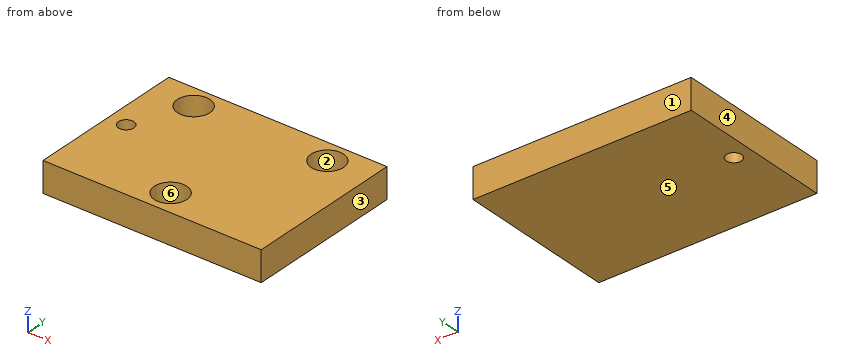
Autodesk Inventor part; units mm, degrees
ref_plane "YZ Plane" through (0, 0, 0) normal (1, 0, 0) x (0, 1, 0)
ref_plane "XZ Plane" through (0, 0, 0) normal (0, 1, 0) x (-1, 0, 0)
ref_plane "XY Plane" through (0, 0, 0) normal (0, 0, 1) x (1, 0, 0)
ref_plane "Work Plane1" through (52.5141, 202.7033, 6.4479) normal (0, 0, -1) x (0, 1, 0)
sketch "Sketch1" plane through (52.5141, 202.7033, 6.4479) normal (0, 0, -1) x (0, 1, 0)
  line L0 (-34.8114, -13.0433) -> (-63.8114, -13.0433)
  line L1 (-63.8114, -13.0433) -> (-63.8114, -52.6244)
  line L2 (-63.8114, -52.6244) -> (-34.8114, -52.6244)
  line L3 (-34.8114, -52.6244) -> (-34.8114, -13.0433)
  circle A0 centre (-59.5444, -32.8338) radius 2.95
  circle A1 centre (-38.8114, -20.7095) radius 2.95
  circle A2 centre (-38.8114, -44.9582) radius 2.95 construction
  line L4 (-60.26, -25.0657) -> (-36.5, -25.0657) construction
  line L5 (-36.5, -25.0657) -> (-36.5, -52.0657) construction
  line L6 (-60.26, -52.0657) -> (-60.26, -25.0657) construction
  line L7 (-57.1632, -22.5233) -> (-33.4032, -22.5233) construction
  line L8 (-33.4032, -22.5233) -> (-33.4032, -49.5233) construction
  line L9 (-33.4032, -49.5233) -> (-57.1632, -49.5233) construction
  line L10 (-57.1632, -49.5233) -> (-57.1632, -22.5233) construction
  circle A3 centre (-38.8114, -44.9582) radius 2.95
  point P0 (-202.7033, -52.5141)
  point P1 (-56.7146, -27.9576)
  point P2 (-25.3114, -32.8338)
  dimension "d4" = 5.9
  dimension "d5" = 5.9
  dimension "d6" = 5.9
  dimension "d37" = 12.1244
  dimension "d38" = 12.1244
extrude "Extrusion1" add sketch "Sketch1" along normal blind 4
sketch "Sketch2" plane through (52.5141, 202.7033, 2.4479) normal (0, 0, -1) x (-1, 0, 0)
  circle A0 centre (44.9582, -38.8114) radius 2.95
  circle A1 centre (20.7095, -38.8114) radius 2.95
  circle A2 centre (32.8338, -59.5444) radius 2.95
  line L0 (13.0433, -34.8114) -> (13.0433, -63.8114)
  line L1 (13.0433, -63.8114) -> (52.6244, -63.8114)
  line L2 (52.6244, -63.8114) -> (52.6244, -34.8114)
  line L3 (52.6244, -34.8114) -> (13.0433, -34.8114)
  point P0 (52.5141, -202.7033)
extrude "Extrusion2" add sketch "Sketch2" along normal blind 1.5 contours A0 | A1 | A2 | L3 L2 L1 L0
sketch "Sketch5" plane through (52.5141, 202.7033, 0.9479) normal (0, 0, -1) x (-1, 0, 0)
  arc A0 (46.5221, -54.1283) -> (46.5221, -43.4579) centre (46.5221, -48.7931) ccw
  circle A1 centre (49.353, -48.7931) radius 1.4
  point P0 (52.5141, -202.7033)
  dimension "d30" = 2.8
extrude "Extrusion5" cut sketch "Sketch5" against normal through all
equation "\"d31\" = d30"
properties part number "cellSTORM_v5_chiptray_old_0"
The listing builds one solid part. Answer for the finished solid, in the listing's coordinates (mm). Face numbers are marked on the shaded views. A direction names the side the tool comes from. Give positions to 0.01 mm unless a question says otherwise; leave off trailing zeros. Write each loop counter-clockwise with the first axis right and the second up, starting at its lowest first coordinate (ties: lowest second). Pieces come first, ordered by that corner, then holes.
1) For a pull along X with two mould halves and no side action, classify the marked faces 1, 2, 3 and 4 as pulls with the +X half, pulls with the -X half, needs draft (parallel to the pull), parting line crosses it, or undercut.
2) Section D-D (y = 164.5) is taken. Write down the section's boundary in (x, z), and give its area (3 significant figures).
3) Section C-C (y = 145.5) is taken. Write down the section's boundary in (x, z), and give its area (3 significant figures).
4) Section A-A (z = 4.85) is taken. Write down the section's boundary in (x, y).
5) Section B-B (x = 32.5) is taken. Write down the section's boundary in (y, z), and give its area (3 significant figures).
6) Find the intervals of material crossed by L1, parallel to X at y = 163.25, z = 3.1; L2, parallel to X at y = 164.75, z = 5.6; L3, parallel to Z at x = 9, y = 163.5, in increasing order.
7) Given P1, Ø3.5, axis at x = 7.56, y = 163.89, coming from the +Z side, flat-ended and moving along its own axis, determine where the tip first touches the part or whether it passes through.
8) A tool of negligible diameter and unlimited length cuts with its end or side. For the marked faces 5 and 6, from which of +Z, -Z, +X, -X, +Y, -Y can it reach the whole face along a straight path? Write none if from no direction.
Response:
1. face 1: needs draft
1. face 2: undercut
1. face 3: pulls with the +X half
1. face 4: pulls with the -X half
2. outline: (-0.11, 0.95) - (39.47, 0.95) - (39.47, 6.45) - (34.69, 6.45) - (34.69, 2.45) - (28.92, 2.45) - (28.92, 6.45) - (10.44, 6.45) - (10.44, 2.45) - (4.67, 2.45) - (4.67, 6.45) - (-0.11, 6.45) - close
2. area: 172 mm2
3. outline: (-0.11, 0.95) - (39.47, 0.95) - (39.47, 6.45) - (21.48, 6.45) - (21.48, 2.45) - (17.89, 2.45) - (17.89, 6.45) - (-0.11, 6.45) - close
3. area: 203 mm2
4. outline: (-0.11, 138.89) - (39.47, 138.89) - (39.47, 167.89) - (-0.11, 167.89) - close; hole circle Ø2.8 at (3.16, 153.91); hole circle Ø5.9 at (7.56, 163.89); hole circle Ø5.9 at (19.68, 143.16); hole circle Ø5.9 at (31.8, 163.89)
5. outline: (138.89, 0.95) - (167.89, 0.95) - (167.89, 6.45) - (166.76, 6.45) - (166.76, 2.45) - (161.03, 2.45) - (161.03, 6.45) - (138.89, 6.45) - close
5. area: 137 mm2
6. L1: x = -0.11 to 4.68, 10.44 to 28.93, 34.68 to 39.47
6. L2: x = -0.11 to 4.73, 10.38 to 28.98, 34.63 to 39.47
6. L3: z = 0.95 to 2.45
7. P1: stops at z = 2.45
8. face 5: -Z, +X, -X, +Y, -Y
8. face 6: +Z
